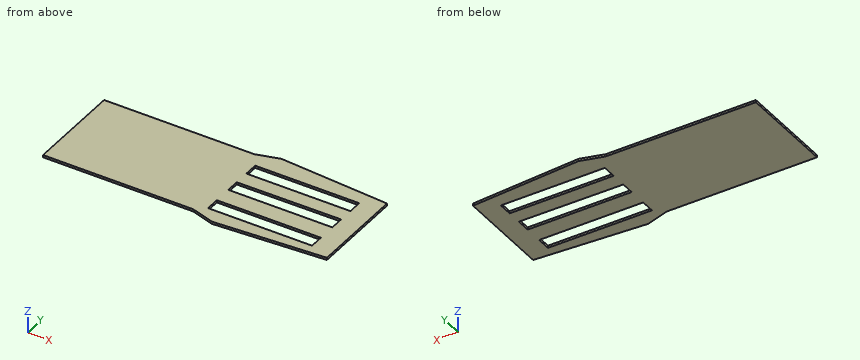
```python
from build123d import *

# Parameters (mm, degrees)
F0_W     = 150
F0_H     = 99
F1_DEPTH = 1
F2_W     = 45
F2_H     = 6
F3_DEPTH = 25


with BuildPart() as f1:
    # F0 (on Top) → F1 (new body)
    with BuildSketch(Plane.XY):
        Rectangle(F0_W, F0_H)
    extrude(amount=F1_DEPTH)

    # F2 (on face) → F3 (cut)
    with BuildSketch(Plane.XY.offset(1)):
        with Locations((16.671137, 13.597774)):
            Rectangle(F2_W, F2_H)
        Polygon((39.171137, -1.737237), (39.171137, 4.262763), (-5.828066, 3.994909), (-5.828066, -1.737237), align=None)
        with Locations((16.671137, -12.613959)):
            Rectangle(F2_W, F2_H)
        Polygon((-75, 49.5), (-75, 22.636687), (-10, 22.636687), (0, 25.437629), (47.867719, 21.876522), (47.911783, -19.269578), (0, -22.178359), (-10, -19.122791), (-75, -19.122791), (-75, -49.5), (75, -49.5), (75, 49.5), align=None)
    extrude(amount=-F3_DEPTH, mode=Mode.SUBTRACT)


solid = f1.part
```
Check sheet for the modelled part. Datum: model origin and axes. Units: mm. Round coordinates to 2 decimals unless told otherwise and drop trailing zeros. Loops run counter-clockwise (first coordinate to the right, second up) from the corner with the lowest first, then second, coordinate; pieces in that order, holes last. Notation, with made-up numbers: (51.25, -30) -> (69.25, -30) arc R16 cw to (69.25, -4) -> close; hole circle Ø7 at (79.5, 2). An arc over 180 degrees is marked (long way). Write item = value, one per line. Start each with the question number.
1) Thickness scan on probe 1 along Y at (x, z) = (5.5, 0.3); probe 2 along Y at (x, z) = (39, 0.6); probe 3 along X at (y, z) = (13, 0.35). Record the ranges inside material, lowest first.
2) Sectioned sample at A-A, the plane z = 0.2. Record the cut outline in (x, y).
3) Sectioned sample at B-B, the plane x = 26.5. Record the cut outline in (y, z).
4) Gauge pin test, flat ends, axial feed: pin 1 Ø5 at (x, y) = (-27, -11) entering from -Z; pin 2 Ø0.5 at (x, z) = (-45, 0.5) entering from -Y. Record the tip position at first contact, or that the pin passes through.
5) Sectioned sample at D-D, the plane x = -12. Record the cut outline in (y, z), plus the area to 3 significant figures.
6) Sectioned sample at C-C, the plane y = 14. Record the cut outline in (x, z), plus the area to 3 significant figures.
Results are:
q1.probe_1 = -21.84 to -15.61, -9.61 to -1.74, 4.06 to 10.6, 16.6 to 25.03
q1.probe_2 = -19.81 to -15.61, -9.61 to -1.74, 4.26 to 10.6, 16.6 to 22.54
q1.probe_3 = -75 to -5.83, 39.17 to 47.88
q2.outline = (-75, -19.12) -> (-10, -19.12) -> (0, -22.18) -> (47.91, -19.27) -> (47.87, 21.88) -> (0, 25.44) -> (-10, 22.64) -> (-75, 22.64) -> close; hole (-5.83, -15.61) -> (39.17, -15.61) -> (39.17, -9.61) -> (-5.83, -9.61) -> close; hole (-5.83, -1.74) -> (39.17, -1.74) -> (39.17, 4.26) -> (-5.83, 3.99) -> close; hole (-5.83, 10.6) -> (39.17, 10.6) -> (39.17, 16.6) -> (-5.83, 16.6) -> close
q3.outline = (-20.57, 0) -> (-15.61, 0) -> (-15.61, 1) -> (-20.57, 1) -> close; (-9.61, 0) -> (-1.74, 0) -> (-1.74, 1) -> (-9.61, 1) -> close; (4.19, 0) -> (10.6, 0) -> (10.6, 1) -> (4.19, 1) -> close; (16.6, 0) -> (23.47, 0) -> (23.47, 1) -> (16.6, 1) -> close
q4.pin_1 = 0
q4.pin_2 = -19.12
q5.outline = (-19.12, 0) -> (22.64, 0) -> (22.64, 1) -> (-19.12, 1) -> close
q5.area = 41.8 mm^2
q6.outline = (-75, 0) -> (-5.83, 0) -> (-5.83, 1) -> (-75, 1) -> close; (39.17, 0) -> (47.88, 0) -> (47.88, 1) -> (39.17, 1) -> close
q6.area = 77.9 mm^2
